Autodesk Inventor part; units mm, degrees
ref_plane "YZ Plane" through (0, 0, 0) normal (1, 0, 0) x (0, 1, 0)
ref_plane "XZ Plane" through (0, 0, 0) normal (0, 1, 0) x (-1, 0, 0)
ref_plane "XY Plane" through (0, 0, 0) normal (0, 0, 1) x (1, 0, 0)
sketch "Sketch1" plane through (0, 0, 0) normal (0, 1, 0) x (-1, 0, 0)
  arc A0 (-110.5448, 1.666) -> (-110.4284, 1.6651) centre (-110.4068, 11.3006) ccw construction
  arc A1 (-94.0784, 1.6651) -> (-94.0348, 1.6644) centre (-93.8968, 11.3006) ccw construction
  circle A2 centre (-110.4068, 11.3006) radius 1.143
  circle A3 centre (-93.8968, 11.3006) radius 1.143
  line L0 (-108.2859, -8.1857) -> (-96.2209, -8.1857) construction
  line L1 (-102.2534, 42.9953) -> (-122.5734, 42.9953)
  line L2 (-102.2534, 42.9953) -> (-81.9334, 42.9953)
  line L3 (-122.5734, 42.9953) -> (-122.5734, -4.3774)
  line L4 (-122.5734, -4.3774) -> (-81.9334, -4.3774)
  line L5 (-81.9334, -4.3774) -> (-81.9334, 42.9953)
  line L6 (-89.5534, -4.3774) -> (-114.9534, -4.3774) construction
  line L7 (-96.0304, 38.4741) -> (-108.4764, 38.4741)
  line L8 (-108.4764, 38.4741) -> (-108.4764, 35.7563)
  line L9 (-108.4764, 35.7563) -> (-96.0304, 35.7563)
  line L10 (-96.0304, 35.7563) -> (-96.0304, 38.4741)
  line L11 (-113.4226, 18.8009) -> (-110.7048, 18.8009)
  line L12 (-110.7048, 18.8009) -> (-110.7048, 31.2469)
  line L13 (-110.7048, 31.2469) -> (-113.4226, 31.2469)
  line L14 (-113.4226, 31.2469) -> (-113.4226, 18.8009)
  line L15 (-91.0842, 18.8009) -> (-93.802, 18.8009)
  line L16 (-93.802, 18.8009) -> (-93.802, 31.2469)
  line L17 (-93.802, 31.2469) -> (-91.0842, 31.2469)
  line L18 (-91.0842, 31.2469) -> (-91.0842, 18.8009)
  arc A4 (-93.8968, 10.028) -> (-93.9768, 12.5706) centre (-93.8968, 11.3006) ccw construction
  arc A5 (-110.3268, 12.5706) -> (-110.4068, 10.028) centre (-110.4068, 11.3006) ccw construction
  line L19 (-109.7718, 18.8653) -> (-94.5318, 18.8653) construction
  line L20 (-91.008, 15.4989) -> (-91.008, 18.6739) construction
  line L21 (-92.4431, 31.2469) -> (-92.4431, 18.8009) construction
  line L22 (-91.0842, 25.0239) -> (-93.802, 25.0239) construction
  line L23 (-112.0637, 18.8009) -> (-112.0637, 31.2469) construction
  line L24 (-110.7048, 25.0239) -> (-113.4226, 25.0239) construction
  line L25 (-96.0304, 37.1152) -> (-108.4764, 37.1152) construction
  line L26 (-102.2534, 35.7563) -> (-102.2534, 38.4741) construction
  point P0 (0, 0)
  point P1 (-102.2534, 36.3575)
  dimension "d0" = 2.286
  dimension "d1" = 2.286
  dimension "d19" = 3.175
  dimension "d23" = 6.223
  dimension "d24" = 1.3589
  dimension "d25" = 6.223
  dimension "d26" = 1.3589
  dimension "d27" = 6.223
  dimension "d28" = 1.3589
extrude "Extrusion1" add sketch "Sketch1" along normal blind 2.921
ref_plane "Work Plane1" through (102.2534, 0, 38.4741) normal (-1, 0, 0) x (0, 0, 1)
sketch "Sketch2" plane through (0, 2.921, 0) normal (0, 1, 0) x (1, 0, 0)
  point P0 (0, 0)
properties part number "arm4_11"
Source: CAD feature listing. Evaluate the final solid. Frame: model axes, mm. A direction names the side the tool comes from. Give positions to 0.01 mm unless a question says otherwise; leave off trailing zeros. Write each loop counter-clockwise with the first axis right and the second up, starting at its lowest first coordinate (ties: lowest second). Pieces come first, ordered by that corner, then holes. Notation, with made-up numbers: M 0,64.5 L 23,64.5 A5 ccw 23,72.5 Z; hole C -7,-34 d3. An arc over 180 degrees is marked long. Return JSON: item names as keys, results as strings. Group by question number.
1) Material intervals for line 1 along X through (y, z) = (1.25, 22); line 2 along X through (y, z) = (2.35, 36.5); line 3 along Z through (x, y) = (92.5, 1), sorted ascending. Write a range as [from, to].
2) Cut plane C-C, the plane y = 1.3. Output: boundary loops of the cut face in (x, z), plus the area to 3 significant figures.
3) Pin query (flat end, axial travel): P1, Ø2, axis at x = 93.9, z = 11.3, coming from the +Y side. Return the tip coordinate at first contact, or that it passes through.
4) Set-up query: faces 4 (the face through (92, 1, 18.801)), 5 (the face through (103, 2.921, 20)). Return all of +Z, -Z, +X, -X, +Y, -Y with unobstructed straight access to the full face (end or side cutting, diameter ignored); none if empty.
5) Cut plane B-B, the plane x = 104. Output: boundary loops of the cut face in (y, z), plus the area to 3 significant figures.
6) Pull-direction query (Z, two-part tool) for faces 1 (the face through (102, 1, 38.474)), 2 (the face through (103, 1, 42.995)), 3 (the face through (81.933, 1, 19)); classes: pulls with the +Z half, pulls with the -Z half, needs draft (parallel to the pull), parting line crosses it, or undercut.
7) Cut plane A-A, the plane z = 27. Output: boundary loops of the cut face in (x, y).
Recorded:
{
 "1": {"line 1": "x = [81.93, 91.08], [93.8, 110.7], [113.42, 122.57]", "line 2": "x = [81.93, 96.03], [108.48, 122.57]", "line 3": "z = [-4.38, 18.8], [31.25, 43]"},
 "2": {"outline": "M 81.93,-4.38 L 122.57,-4.38 L 122.57,43 L 81.93,43 Z; hole M 91.08,18.8 L 93.8,18.8 L 93.8,31.25 L 91.08,31.25 Z; hole C 93.9,11.3 d2.29; hole M 96.03,35.76 L 108.48,35.76 L 108.48,38.47 L 96.03,38.47 Z; hole C 110.41,11.3 d2.29; hole M 110.7,18.8 L 113.42,18.8 L 113.42,31.25 L 110.7,31.25 Z", "area": "1,820 mm²"},
 "3": {"P1": "passes through"},
 "4": {"face 4": "+Y, -Y", "face 5": "+Z, -Z, +X, -X, +Y"},
 "5": {"outline": "M 0,-4.38 L 2.92,-4.38 L 2.92,35.76 L 0,35.76 Z; M 0,38.47 L 2.92,38.47 L 2.92,43 L 0,43 Z", "area": "130 mm²"},
 "6": {"face 1": "undercut", "face 2": "pulls with the +Z half", "face 3": "needs draft"},
 "7": {"outline": "M 81.93,0 L 91.08,0 L 91.08,2.92 L 81.93,2.92 Z; M 93.8,0 L 110.7,0 L 110.7,2.92 L 93.8,2.92 Z; M 113.42,0 L 122.57,0 L 122.57,2.92 L 113.42,2.92 Z"}
}
